Can you work these out from the model? Positions are in its coordinate system, mm. Face numbers are marked on the shaded views. A direction names the side the tool comes from. Round coordinates to 2 decimals unless told otherwise and drop trailing zeros. Order: outer loops, then holes, each group sorted by start corner. A loop starts at its lowest first (then second) coordinate and runs counter-clockwise, first axis right, second up.
Q1. If we section it at C-C (y = 4.4): Please give me the cut outline in (x, z).
Q2. Will these pins go through, and if not, where does the flat tip stop? P1, Ø3, axis at x = -24.55, z = 29, coming from the -Y side; P2, Ø1.6, axis at x = -25, y = 0.5, coming from the +Z side; P3, Ø5, axis at x = -24.55, z = -29, coming from the +Y side; P4, Ø1.6, axis at x = -22.5, y = 0.5, coming from the -Z side.
Q3. If we section it at D-D (x = -4): Please give me the cut outline in (y, z).
Q4. If we section it at A-A (x = -24.55): Please give me the cut outline in (y, z), plus the area to 3 significant figures.
Q5. For the marked faces 1 and 2, which set-ups out of +Z, -Z, +X, -X, +Y, -Y let a thin tool reach every point of the face, with its end or its side?
Q6. If I drill on line 1 (Z direction, x = -24.55, y = 0.9); line 2 (X direction, y = 0.65, z = 29); line 3 (Z direction, x = -6.5, y = 3.5), over which ranges is the centre line in solid material (lowest first)?
Q7. If we section it at B-B (z = 29): Please give me the cut outline in (x, y), plus the area to 3 significant figures.
Autodesk Inventor part; units mm, degrees
ref_plane "YZ Plane" through (0, 0, 0) normal (1, 0, 0) x (0, 1, 0)
ref_plane "XZ Plane" through (0, 0, 0) normal (0, 1, 0) x (-1, 0, 0)
ref_plane "XY Plane" through (0, 0, 0) normal (0, 0, 1) x (1, 0, 0)
sketch "Boceto1" plane through (0, 0, 0) normal (0, 1, 0) x (-1, 0, 0)
  line L0 (-19, -70.5) -> (19, -70.5)
  line L1 (19, -70.5) -> (19, 70.5)
  line L2 (19, 70.5) -> (-19, 70.5)
  line L3 (-19, 70.5) -> (-19, -70.5)
  line L4 (-19, -70.5) -> (19, 70.5) construction
  line L5 (19, -70.5) -> (-19, 70.5) construction
  line L6 (-30, -35) -> (30, -35)
  line L7 (30, -35) -> (30, 35)
  line L8 (30, 35) -> (-30, 35)
  line L9 (-30, 35) -> (-30, -35)
  line L10 (-30, -35) -> (30, 35) construction
  line L11 (30, -35) -> (-30, 35) construction
  point P0 (0, 0)
  point P1 (-19, 35)
  point P2 (-19, -35)
  point P3 (19, -35)
  point P4 (19, 35)
  dimension "d0" = 141
  dimension "d1" = 38
  dimension "d2" = 70
  dimension "d3" = 60
extrude "Extrusión1" add sketch "Boceto1" along normal blind 1.5
sketch "Boceto2" plane through (0, 1.5, 0) normal (0, 1, 0) x (1, 0, 0)
  line L0 (24.55, 29) -> (-24.55, 29)
  line L1 (-24.55, 29) -> (-24.55, -29)
  line L2 (-24.55, -29) -> (24.55, -29)
  line L3 (24.55, -29) -> (24.55, 29)
  line L4 (24.55, 29) -> (-24.55, -29) construction
  line L5 (-24.55, 29) -> (24.55, -29) construction
  point P0 (0, 0)
  dimension "d6" = 49.1
  dimension "d7" = 58
hole "Agujero1" at (-24.55, 1.5, 29) at (-24.55, 1.5, -29) at (24.55, 1.5, -29) at (24.55, 1.5, 29) direction (0, -1, 0) diameter 3.1 end through all
sketch "Boceto3" plane through (0, 1.5, 0) normal (0, 1, 0) x (1, 0, 0)
  line L0 (-19, -35) -> (-19, -70.5)
  line L1 (19, -70.5) -> (19, -35)
  line L2 (-19, -70.5) -> (19, -70.5)
  line L3 (19, -70.5) -> (19, -69)
  line L4 (19, -69) -> (-19, -69)
  line L5 (-19, -69) -> (-19, -70.5)
  point P0 (0, 0)
  point P1 (19, -70.5)
  dimension "d15" = 1.5
extrude "Extrusión2" add sketch "Boceto3" along normal blind 4
mirror "Simetría1" about plane through (0, 0, 0) normal (0, 0, 1) of "Extrusión2"
properties part number "Soporte_bateria_p1_3DPrint"
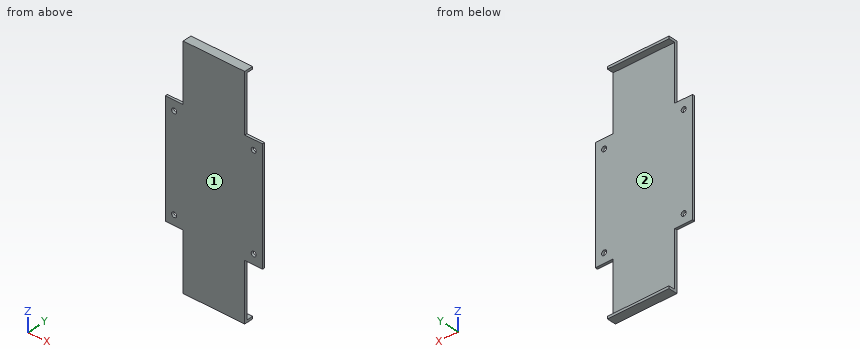
Solution:
1. outline: (-19, -70.5) - (19, -70.5) - (19, -69) - (-19, -69) - close; (-19, 69) - (19, 69) - (19, 70.5) - (-19, 70.5) - close
2. P1: passes through
2. P2: stops at z = 35
2. P3: stops at y = 1.5
2. P4: stops at z = -35
3. outline: (0, -70.5) - (5.5, -70.5) - (5.5, -69) - (1.5, -69) - (1.5, 69) - (5.5, 69) - (5.5, 70.5) - (0, 70.5) - close
4. outline: (0, -35) - (1.5, -35) - (1.5, -30.55) - (0, -30.55) - close; (0, -27.45) - (1.5, -27.45) - (1.5, 27.45) - (0, 27.45) - close; (0, 30.55) - (1.5, 30.55) - (1.5, 35) - (0, 35) - close
4. area: 95.7 mm2
5. face 1: +Z, -Z, +X, -X, -Y
5. face 2: +X, -X, +Y
6. line 1: z = -35 to -30.55, -27.45 to 27.45, 30.55 to 35
6. line 2: x = -30 to -26.1, -23 to 23, 26.1 to 30
6. line 3: z = -70.5 to -69, 69 to 70.5
7. outline: (-30, 0) - (-26.1, 0) - (-26.1, 1.5) - (-30, 1.5) - close; (-23, 0) - (23, 0) - (23, 1.5) - (-23, 1.5) - close; (26.1, 0) - (30, 0) - (30, 1.5) - (26.1, 1.5) - close
7. area: 80.7 mm2
